The model under review builds one solid part; all positions refer to its coordinate system, in mm. A direction names the side the tool comes from. Coordinates: 2 decimals unless noted, no trailing zeros. Write each loop counter-clockwise with the first axis right and the second up, starting at its lowest first coordinate (ties: lowest second). Pieces come first, ordered by that corner, then holes. Notation, with made-up numbers: (16, -29) - (36, -29) arc R20 cw to (36, -23) - close; hole circle Ø10 at (33, 29). An arc over 180 degrees is marked (long way). Put each result on its own line as item: value. Start each with the question number.
Item 1: For pin 1 (8 mm diameter, centred on x = -9, z = -6, fed in from +Y); pin 2 (0.8 mm diameter, centred on y = -13, z = -6.5, fed in from +X); pin 3 (2.5 mm diameter, centred on x = -14.5, z = -1.5, fed in from +Y), all flat-tipped, find the tip position at first contact; note any pin that passes through.
Item 2: To check wall thickness, follow L1, parallel to Z at x = -11, y = -6.5; L2, parallel to Y at x = -12.5, z = -0.5; L3, parallel to X at y = 5.5, z = -1.75. State the ranges of each line that lie inside material, in increasing order. Write a range as [from, to].
Item 3: Consider section A-A on z = -2.5. Give the boundary of the cut face in (x, y).
Item 4: Consider section D-D on z = -9. Give the boundary of the cut face in (x, y), then the cut area to 3 significant figures.
Item 5: Mouldability with a two-part tool opening along Y and no side actions: class faces 1 (the face through (21.36, -9.76, -6.88)), 2 (the face through (12.8, 6.5, -6.9)), 3 (the face through (20.73, -9.4, -1.58)), 4 (the face through (11, 8, 0)) as pulls with the +Y half, pulls with the -Y half, needs draft (parallel to the pull), parting line crosses it, or undercut.
Item 6: Machinability: for faces 5 (the face through (-21.47, -9.65, -6.88)), 6 (the face through (0, -13, -11.8)), 7 (the face through (11.71, 5.47, -8.04)), which of the approach directions +Z, -Z, +X, -X, +Y, -Y give a long, thin tool a straight path to every point of the face, cutting with its end or side? Answer none if there is none.
Item 7: Consider section B-B on y = 1. Give the boundary of the cut face in (x, z).
Item 8: Consider section C-C on x = 19. Give the boundary of the cut face in (y, z).
```python
from build123d import *

# Parameters (mm, degrees)
EXTRUDE_1_DEPTH          = 12.75
EXTRUDE_1_DEPTH_BACK     = 12.75
EXTRUDE_1_2_DEPTH        = 1.2
EXTRUDE_2_DEPTH          = 1.2
SKETCH_4_W               = 23.6
SKETCH_4_H               = 23.6
CUT_EXTRUDE_1_DEPTH      = 1.5
CUT_EXTRUDE_2_DEPTH      = 35.680906203
CUT_EXTRUDE_2_DEPTH_BACK = 35.680906203
SKETCH_5_W               = 13.95
SKETCH_5_H               = 32.801494515
CUT_EXTRUDE_3_DEPTH      = 3.2


with BuildPart() as part:
    # Эскиз1 → Extrude 1 (new, two sides: drawn at the far end of the back side and taken through both)
    with BuildSketch(Plane.XY.offset(-EXTRUDE_1_DEPTH_BACK)):
        Polygon((-17.621320344, -13.5), (17.621320344, -13.5), (25.211407429, -5.909912914), (0, 19.301494515), (-25.211407429, -5.909912914), align=None)
        Polygon((-17, -12), (17, -12), (23.090087086, -5.909912914), (0, 17.180174171), (-23.090087086, -5.909912914), align=None, mode=Mode.SUBTRACT)
    extrude(amount=EXTRUDE_1_DEPTH + EXTRUDE_1_DEPTH_BACK)

    # Эскиз2 → Extrude 1 2 (add)
    with BuildSketch(Plane.XY.offset(12.75)):
        Polygon((25.211407429, -5.909912914), (0, 19.301494515), (-25.211407429, -5.909912914), (-17.621320344, -13.5), (17.621320344, -13.5), align=None)
    extrude(amount=EXTRUDE_1_2_DEPTH)

    # Эскиз3 → Бобышка-Вытянуть2 (add)
    with BuildSketch(Plane(origin=(0, 0, -12.75), x_dir=(-1, 0, 0), z_dir=(0, 0, -1))):
        Polygon((0, 19.301494515), (25.211407429, -5.909912914), (17.621320344, -13.5), (-17.621320344, -13.5), (-25.211407429, -5.909912914), align=None)
    extrude(amount=EXTRUDE_2_DEPTH)

    # Эскиз4 → Вырез-Вытянуть1 (cut)
    with BuildSketch(Plane.XZ.offset(13.5)):
        Rectangle(SKETCH_4_W, SKETCH_4_H)
    extrude(amount=-CUT_EXTRUDE_1_DEPTH, mode=Mode.SUBTRACT)

    # Эскиз5 → Вырез-Вытянуть2 (cut, two sides: drawn at the far end of the back side and taken through both)
    with BuildSketch(Plane(origin=(0, 0, 0), x_dir=(0, 0, -1), z_dir=(1, 0, 0)).offset(-CUT_EXTRUDE_2_DEPTH_BACK)):
        with Locations((-6.975, 2.900747258)):
            Rectangle(SKETCH_5_W, SKETCH_5_H)
    extrude(amount=CUT_EXTRUDE_2_DEPTH + CUT_EXTRUDE_2_DEPTH_BACK, mode=Mode.SUBTRACT)

    # Эскиз6 → Вырез-Вытянуть3 (cut)
    with BuildSketch(Plane.XY):
        Polygon((-17.33137085, -12.8), (17.33137085, -12.8), (24.221457935, -5.909912914), (0, 18.311545021), (-24.221457935, -5.909912914), align=None)
    extrude(amount=-CUT_EXTRUDE_3_DEPTH, mode=Mode.SUBTRACT)


solid = part.part
```
Report:
1. pin 1: y = 14.3
1. pin 2: x = 18.52
1. pin 3: y = 6.05
2. L1: [-13.95, -12.75]
2. L2: [-13.5, -12.8], [5.81, 6.8]
2. L3: [-13.8, -12.81], [12.81, 13.8]
3. outline: (-25.21, -5.91) - (-17.62, -13.5) - (-11.8, -13.5) - (-11.8, -12.8) - (-17.33, -12.8) - (-24.22, -5.91) - (0, 18.31) - (24.22, -5.91) - (17.33, -12.8) - (11.8, -12.8) - (11.8, -13.5) - (17.62, -13.5) - (25.21, -5.91) - (0, 19.3) - close
4. outline: (-25.21, -5.91) - (-17.62, -13.5) - (-11.8, -13.5) - (-11.8, -12) - (-17, -12) - (-23.09, -5.91) - (0, 17.18) - (23.09, -5.91) - (17, -12) - (11.8, -12) - (11.8, -13.5) - (17.62, -13.5) - (25.21, -5.91) - (0, 19.3) - close
4. area: 148 mm²
5. face 1: pulls with the -Y half
5. face 2: pulls with the +Y half
5. face 3: undercut
5. face 4: needs draft
6. face 5: +Z, -Z, -X, -Y
6. face 6: +Z, -Y
6. face 7: +Z
7. outline: (-18.3, -13.95) - (18.3, -13.95) - (18.3, 0) - (17.31, 0) - (17.31, -3.2) - (16.18, -3.2) - (16.18, -12.75) - (-16.18, -12.75) - (-16.18, -3.2) - (-17.31, -3.2) - (-17.31, 0) - (-18.3, 0) - close
8. outline: (-12.12, -13.95) - (0.3, -13.95) - (0.3, 0) - (-0.69, 0) - (-0.69, -3.2) - (-1.82, -3.2) - (-1.82, -12.75) - (-10, -12.75) - (-10, -3.2) - (-11.13, -3.2) - (-11.13, 0) - (-12.12, 0) - close
